Input: part model. Units: mm. Frame: model coordinates. A direction names the side the tool comes from. Give positions to 0.01 mm unless a question says otherwise; leave off trailing zeros. Order: outer loops, then holes, each group sorted by start corner. A loop starts at its lowest first (then second) coordinate and runs counter-clockwise, first axis right, second up. Notation, with made-up numbers: (-16.5, -36) - (9.5, -36) arc R29 cw to (9.5, 2) - close; hole circle Ø8 at (48.5, -21.75). An arc over 180 degrees is marked (long way). Use a Markdown table: item, result.
from build123d import *

# Parameters (mm, degrees)
F0_R     = 11.735047
F1_DEPTH = 7.366
F2_R     = 4.292472
F3_R     = 5.7912
F4_DEPTH = 0.762
F5_R     = 1.875011
F6_DEPTH = 40.64


with BuildPart() as f1:
    # F0 (on Top) → F1 (new body)
    with BuildSketch(Plane.XY):
        Circle(F0_R)
    extrude(amount=F1_DEPTH)

    # F2
    f2_edges = [f1.edges().sort_by_distance(p)[0] for p in [
        (-11.735047, 0, 7.366),
    ]]
    fillet(f2_edges, radius=F2_R)

    # F3 (on face) → F4 (cut)
    with BuildSketch(Plane(origin=(0, 0, 0), x_dir=(1, 0, 0), z_dir=(0, 0, -1))):
        Circle(F3_R)
    extrude(amount=-F4_DEPTH, mode=Mode.SUBTRACT)

    # F5 (on Front) → F6 (join)
    with BuildSketch(Plane.XZ):
        with Locations((0, 3.073911)):
            Circle(F5_R)
    extrude(amount=F6_DEPTH)


solid = f1.part
1. Pin query (flat end, axial travel): pin 1 (10.5 mm diameter, centred on x = 0, y = 0, fed in from -Z); pin 2 (1.5 mm diameter, centred on x = 6.5, y = -11.5, fed in from +Z); pin 3 (3 mm diameter, centred on y = -18.5, z = 2, fed in from -X) (3 decimals); pin 4 (3 mm diameter, centred on x = 6.5, z = 3.5, fed in from -Y). Return the tip coordinate at first contact, or that it passes through.
Response:
| item | result |
|---|---|
| pin 1 | stops at z = 0.76 |
| pin 2 | passes through |
| pin 3 | stops at x = -1.875 |
| pin 4 | stops at y = -10.6 |
2. Section query C-C (z = 5.5). Return loops of the section in (x, y), then the cut area to 3 significant figures.
Response:
| item | result |
|---|---|
| outline | circle Ø21.97 at (0, 0) |
| area | 379 mm^2 |
3. Material intervals for line 1 along X through (y, z) = (0, 0.4); line 2 along Z through (x, y) = (0.25, 0.5), sorted ascending.
Response:
| item | result |
|---|---|
| line 1 | x = -11.74 to -5.79, 5.79 to 11.74 |
| line 2 | z = 0.76 to 7.37 |
4. Set-up query: faces 5 (the face through (0, 0, 7.366)), 6 (the face through (1.8, -25.8, 3.6)). Return all of +Z, -Z, +X, -X, +Y, -Y with unobstructed straight access to the full face (end or side cutting, diameter ignored); none if empty.
Response:
| item | result |
|---|---|
| face 5 | +Z, +X, -X, +Y, -Y |
| face 6 | -Y |
5. Section query B-B (x = 0). Return loops of the section in (y, z), then the cut area to 3 significant figures.
Response:
| item | result |
|---|---|
| outline | (-40.64, 1.2) - (-11.74, 1.2) - (-11.74, 0) - (-5.79, 0) - (-5.79, 0.76) - (5.79, 0.76) - (5.79, 0) - (11.74, 0) - (11.74, 3.07) arc R4.29 ccw to (7.44, 7.37) - (-7.44, 7.37) arc R4.29 ccw to (-11.3, 4.95) - (-40.64, 4.95) - close |
| area | 265 mm^2 |
6. Section query D-D (y = -33.5). Return loops of the section in (x, z), then the cut area to 3 significant figures.
Response:
| item | result |
|---|---|
| outline | circle Ø3.75 at (0, 3.07) |
| area | 11.0 mm^2 |
7. Section query A-A (y = 0). Return loops of the section in (x, z), then the cut area to 3 significant figures.
Response:
| item | result |
|---|---|
| outline | (-11.74, 0) - (-5.79, 0) - (-5.79, 0.76) - (5.79, 0.76) - (5.79, 0) - (11.74, 0) - (11.74, 3.07) arc R4.29 ccw to (7.44, 7.37) - (-7.44, 7.37) arc R4.29 ccw to (-11.74, 3.07) - close |
| area | 156 mm^2 |
8. Mould query, pull axis X, two halves, no side actions, for faces 1 (the face through (0, 0, 0.762)), 2 (the face through (-2.544, -11.456, 1.515)), 3 (the face through (0, -40.64, 3)), 4 (the face through (-1.255, 5.653, 0.376)). Classes: pulls with the +X half, pulls with the -X half, needs draft (parallel to the pull), parting line crosses it, or undercut.
Response:
| item | result |
|---|---|
| face 1 | undercut |
| face 2 | parting line crosses it |
| face 3 | needs draft |
| face 4 | undercut |
